For this review, use the dimensioned drawing (mm, ordinates from the lowest corner) and the shaded views. Coordinates: 2 decimals unless noted, no trailing zeros. Write each loop counter-clockwise with the first axis right and the second up, starting at its lowest first coordinate (ties: lowest second). Pieces come first, ordered by that corner, then holes. Notation, with made-up numbers: M 10.5,88.25 L 51.5,88.25 A28 ccw 51.5,119.25 Z; hole C 59,-6 d7. An arc over 180 degrees is marked long. Return JSON: item names as keys, results as strings.
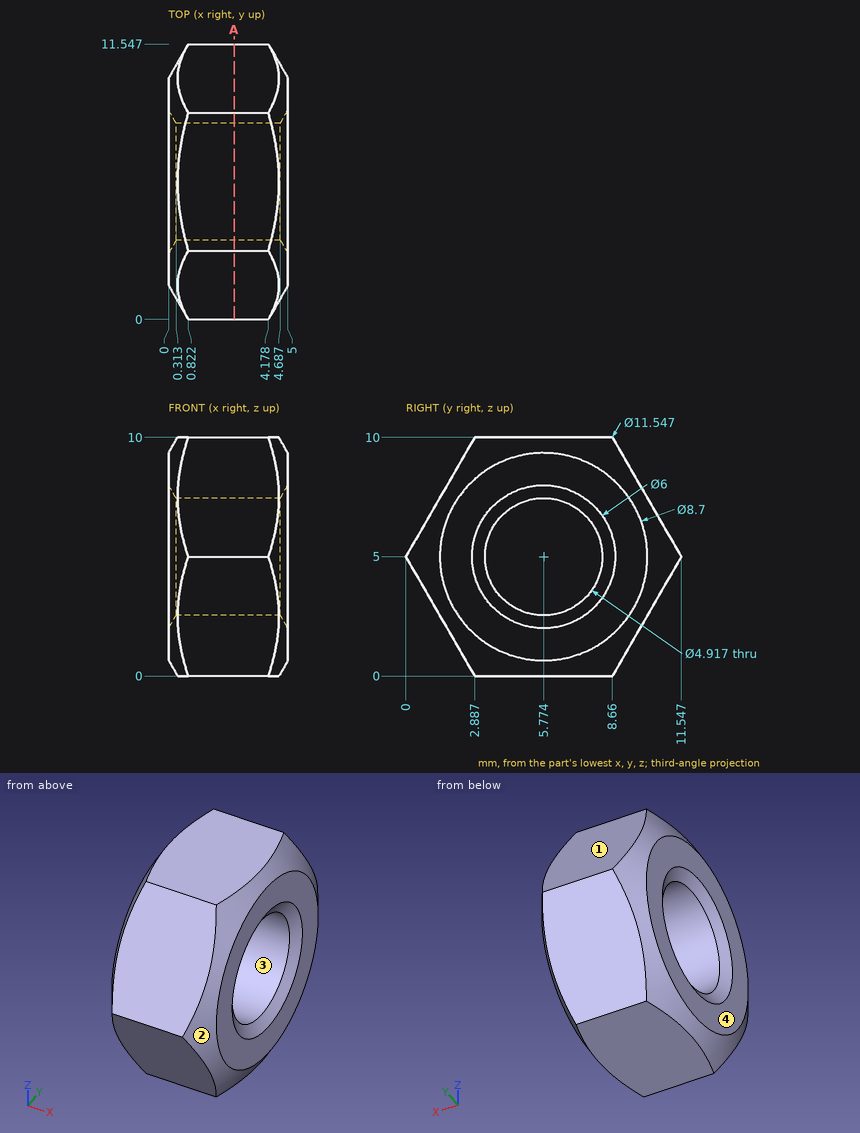
1. Clearance check with a flat-ended pin moving along its axis: pin 1 Ø4.5 at (y, z) = (5.77, 5) entering from +X. State where the tip first meets the part, or that it passes through.
Checks:
{"pin 1": "through"}
2. We need section A-A (x = 2.75). State the section outline as (y, z) points.
Checks:
{"outline": "M 0,5 L 2.89,0 L 8.66,0 L 11.55,5 L 8.66,10 L 2.89,10 Z; hole C 5.77,5 d4.92"}
3. Wall thickness on L1, parallel to Z at x = 1.75, y = 7.75 (1 decimal); L2, parallel to Z at x = 2.4, y = 4.5 (1 decimal); L3, parallel to Z at x = 3.7, y = 9 (1 decimal): over which ranges is each line inside the solid? List them lowest first. Write a range as from..to.
Checks:
{"L1": "0..3.5, 6.5..10", "L2": "0..2.9, 7.1..10", "L3": "0.6..9.4"}
4. Draft analysis for pull direction Z (two halves, no side actions). For the marked faces 1, 2, 3 and 4, state which applies: +Z half, -Z half, draft (parallel to the pull), parting line (faces both ways), or undercut.
Checks:
{"face 1": "+Z half", "face 2": "parting line", "face 3": "undercut", "face 4": "draft"}
